Could you check a few things on this model? Use its own coordinates, in mm. Coordinates: 2 decimals unless noted, no trailing zeros. Order: outer loops, then holes, each group sorted by start corner. A loop starts at its lowest first (then second) coordinate and runs counter-clockwise, first axis right, second up. Notation, with made-up numbers: (50.25, 70) - (107.25, 70) arc R24 ccw to (107.25, 103) - close; hole circle Ø3 at (26.25, 27.25). An arc over 180 degrees is marked (long way). Answer as a JSON object with one key per item and string values. Group by question number.
(1) Please list where these lines run through material, in increasing order: probe 1 along Y at (x, z) = (-3.75, 0.1); probe 2 along Z at (x, y) = (0.25, -0.85).
(2) Imagine slicing it at A-A, the plane x = 6.5. Write out the boundary of the cut face in (y, z).
(3) Will this pin go through, and if not, where does the flat tip stop? P1, Ø2, axis at x = -7.5, y = -1.5, coming from the +Z side.
from build123d import *

# Parameters (mm, degrees)
SKETCH2_R           = 2
EXTRUDE1_DEPTH      = 9.37
EXTRUDE1_DEPTH_BACK = 9.37
SKETCH3_R           = 2
EXTRUDE2_DEPTH      = 0.63
EXTRUDE2_TAPER      = 15
SKETCH4_R           = 2
EXTRUDE3_DEPTH      = 0.63
EXTRUDE3_TAPER      = 15


with BuildPart() as part:
    # Sketch2 → Extrude1 (new body, two sides)
    with BuildSketch(Plane(origin=(0, 0, 0), x_dir=(0, 0, -1), z_dir=(1, 0, 0))) as extrude1_sk:
        Circle(SKETCH2_R)
    extrude(amount=EXTRUDE1_DEPTH)
    extrude(extrude1_sk.sketch, amount=-EXTRUDE1_DEPTH_BACK)

    # Sketch3 → Extrude2 (add)
    with BuildSketch(Plane(origin=(9.37, 0, 0), x_dir=(0, 0, -1), z_dir=(1, 0, 0))):
        Circle(SKETCH3_R)
    extrude(amount=EXTRUDE2_DEPTH, taper=EXTRUDE2_TAPER)

    # Sketch4 → Extrude3 (add)
    with BuildSketch(Plane.ZY.offset(9.37)):
        Circle(SKETCH4_R)
    extrude(amount=EXTRUDE3_DEPTH, taper=EXTRUDE3_TAPER)


solid = part.part
Result set:
{
 "1": {"probe 1": "y = -2 to 2", "probe 2": "z = -1.81 to 1.81"},
 "2": {"outline": "circle Ø4 at (0, 0)"},
 "3": {"P1": "stops at z = 1.94"}
}
